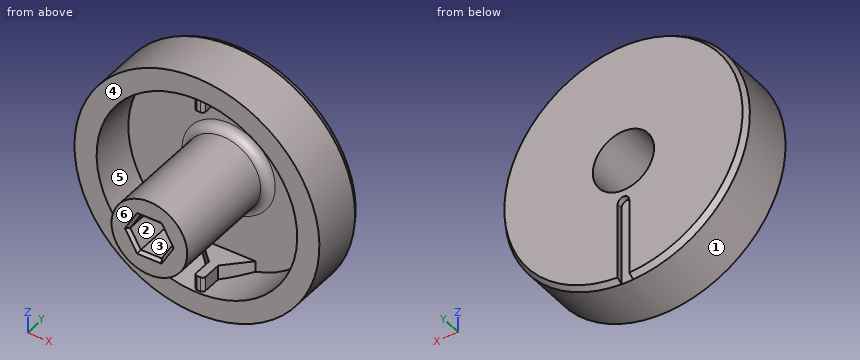
from build123d import *
from build123d.topology import SkipClean

# Parameters (mm, degrees)
SKETCH1_R           = 10.5
SKETCH1_R_2         = 8.6
BOSS_EXTRUDE1_DEPTH = 4
BOSS_EXTRUDE2_DEPTH = 1.25
BOSS_EXTRUDE3_START = 17.2
BOSS_EXTRUDE3_DEPTH = 1.25
BOSS_EXTRUDE4_START = 1
SKETCH3_R           = 10.5
BOSS_EXTRUDE4_DEPTH = 1
SKETCH5_R           = 3.25
BOSS_EXTRUDE5_DEPTH = 10
FILLET2_R           = 0.75
CUT_EXTRUDE1_DEPTH  = 5.25
FILLET1_R           = 0.25
SKETCH7_R           = 2.625
CUT_EXTRUDE2_DEPTH  = 2
CUT_EXTRUDE3_DEPTH  = 0.5
CUT_EXTRUDE4_DEPTH  = 4
CHAMFER2_SIZE       = 0.25
CHAMFER3_SIZE       = 0.5
CHAMFER3_SIZE2      = 0.288675135


with BuildPart() as part:
    # Sketch1 → Boss-Extrude1 (new body)
    with BuildSketch(Plane(origin=(0, 0, 0), x_dir=(1, 0, 0), z_dir=(0, 1, 0))):
        with Locations(Location((0, 0, 0), (0, 0, 270))):
            Circle(SKETCH1_R)
        with Locations(Location((0, 0, 0), (0, 0, 270))):
            Circle(SKETCH1_R_2, mode=Mode.SUBTRACT)
    extrude(amount=-BOSS_EXTRUDE1_DEPTH)

    # Sketch2 → Boss-Extrude2 (add)
    with BuildSketch(Plane(origin=(0, 0, 8.6), x_dir=(-1, 0, 0), z_dir=(0, 0, -1))):
        Polygon((0.4, -3.75), (-0.4, -3.75), (-0.4, -1.9), (-2.3, 0), (2.3, 0), (0.4, -1.9), align=None)
    extrude(amount=BOSS_EXTRUDE2_DEPTH)

    # Sketch2<2> → Boss-Extrude3 (add)
    with BuildSketch(Plane(origin=(0, 0, 8.6), x_dir=(-1, 0, 0), z_dir=(0, 0, -1)).offset(BOSS_EXTRUDE3_START)):
        Polygon((0.4, -3.75), (-0.4, -3.75), (-0.4, -1.9), (-2.3, 0), (2.3, 0), (0.4, -1.9), align=None)
    extrude(amount=-BOSS_EXTRUDE3_DEPTH)

    # Sketch3 → Boss-Extrude4 (add)
    with BuildSketch(Plane(origin=(0, 0, 0), x_dir=(1, 0, 0), z_dir=(0, 1, 0)).offset(BOSS_EXTRUDE4_START)):
        with Locations(Location((0, 0, 0), (0, 0, 270))):
            Circle(SKETCH3_R)
    extrude(amount=-BOSS_EXTRUDE4_DEPTH)

    # Sketch5 → Boss-Extrude5 (add)
    with BuildSketch(Plane.XZ):
        with Locations(Location((0, 0, 0), (0, 0, 90))):
            Circle(SKETCH5_R)
    extrude(amount=BOSS_EXTRUDE5_DEPTH)

    # Fillet2
    fillet2_edges = [part.edges().sort_by_distance(p)[0] for p in [
        (0, 0, -3.25),
    ]]
    fillet(fillet2_edges, radius=FILLET2_R)

    # Sketch4 → Cut-Extrude1 (cut)
    with BuildSketch(Plane(origin=(0, 1, 0), x_dir=(1, 0, 0), z_dir=(0, 1, 0))):
        with BuildLine():
            Line((-1.469693846, 2.175), (1.469693846, 2.175))
            ThreePointArc((1.469693846, 2.175), (0, -2.625), (-1.469693846, 2.175))
        make_face()
    extrude(amount=-CUT_EXTRUDE1_DEPTH, mode=Mode.SUBTRACT)

    # Fillet1
    fillet1_edges = [part.edges().sort_by_distance(p)[0] for p in [
        (-0.4, -3.75, 7.970346319),
        (0.4, -3.75, 7.970346319),
        (-0.4, -3.75, -7.970346319),
        (0.4, -3.75, -7.970346319),
    ]]
    fillet(fillet1_edges, radius=FILLET1_R)

    # Sketch7 → Cut-Extrude2 (cut)
    with SkipClean():  # the faces are left unmerged after this step: merging them gives an invalid solid
        with BuildSketch(Plane(origin=(0, 1, 0), x_dir=(1, 0, 0), z_dir=(0, 1, 0))):
            with Locations(Location((0, 0, 0), (0, 0, 270))):
                Circle(SKETCH7_R)
        extrude(amount=-CUT_EXTRUDE2_DEPTH, mode=Mode.SUBTRACT)

    # Sketch9 → Cut-Extrude3 (cut)
    with SkipClean():  # the faces are left unmerged after this step: merging them gives an invalid solid
        with BuildSketch(Plane(origin=(0, 1, 0), x_dir=(1, 0, 0), z_dir=(0, 1, 0))):
            with BuildLine():
                Line((-0.5, 3.7), (-0.5, 13.7))
                ThreePointArc((-0.5, 13.7), (0, 14.2), (0.5, 13.7))
                Line((0.5, 13.7), (0.5, 3.7))
                ThreePointArc((0.5, 3.7), (0, 3.2), (-0.5, 3.7))
            make_face()
        extrude(amount=-CUT_EXTRUDE3_DEPTH, mode=Mode.SUBTRACT)

    # Sketch10 → Cut-Extrude4 (cut)
    with SkipClean():  # the faces are left unmerged after this step: merging them gives an invalid solid
        with BuildSketch(Plane.XZ.offset(10)):
            Polygon((1.804219591, 0), (0.902109796, 1.5625), (-0.902109796, 1.5625), (-1.804219591, 0), (-0.902109796, -1.5625), (0.902109796, -1.5625), align=None)
        extrude(amount=-CUT_EXTRUDE4_DEPTH, mode=Mode.SUBTRACT)

    # Chamfer2
    chamfer2_edges = [part.edges().sort_by_distance(p)[0] for p in [
        (1.353164693, -10, -0.78125),
        (1.353164693, -10, 0.78125),
        (0, -10, 1.5625),
        (-1.353164693, -10, 0.78125),
        (-1.353164693, -10, -0.78125),
        (0, -10, -1.5625),
    ]]
    chamfer(chamfer2_edges, length=CHAMFER2_SIZE)

    # Chamfer3
    chamfer3_edges = [part.edges().sort_by_distance(p)[0] for p in [
        (-10.497021698, 1, 0.250070932),
    ]]
    chamfer3_side = [part.faces().sort_by_distance(p)[0] for p in [
        (0, -1.5, -10.5),
    ]]
    chamfer(chamfer3_edges, length=CHAMFER3_SIZE, length2=CHAMFER3_SIZE2, reference=chamfer3_side[0])


solid = part.part
Can you work these out from the model? Positions are in its coordinate system, mm. Face numbers are marked on the shaded views. A direction names the side the tool comes from. Coordinates: 2 decimals unless noted, no trailing zeros. Order: outer loops, then holes, each group sorted by start corner. A loop starts at its lowest first (then second) coordinate and runs counter-clockwise, first axis right, second up. Notation, with made-up numbers: (-30.75, -14) - (-9.75, -14) arc R16 ccw to (-9.75, -1) - close; hole circle Ø8 at (71.25, 18.5). An arc over 180 degrees is marked (long way). Answer as a JSON object with one key per item and string values. Group by question number.
Q1. On a 3-axis mill with a long thin cutter (end or side, diameter ignored), from which of +Z, -Z, +X, -X, +Y, -Y can I reach the whole of each face in a straight line? I mean the marked faces 5 and 6. Say none if no direction works.
Q2. Will these pins go through, and if not, where does the flat tip stop? P1, Ø2.5, axis at x = 0, z = 0, coming from the -Y side; P2, Ø0.9, axis at x = -0.5, y = -7.5, coming from the -Z side; P3, Ø0.6, axis at y = 1, z = -6.5, coming from the -X side.
Q3. I need wall thicknesses on line 1 (X direction, y = -2.75, z = 0) (3 decimals); line 2 (X direction, y = -3.25, z = -7.5); line 3 (Y direction, x = 3.5, z = -7.5). Which ranges of each line are inside material? Lowest first, please. Write a range as from..to.
Q4. Imagine slicing it at A-A (y = -8). Please give me the cut outline in (x, z), and give its area (3 significant figures).
Q5. We'd pull the mould along Z, two halves only. Please class the marked faces 1, 2, 3 and 4: +Z half, -Z half, draft (parallel to the pull), parting line (faces both ways), or undercut.
Determined:
{
 "1": {"face 5": "-Y", "face 6": "+Z, -Z, +X, -X, -Y"},
 "2": {"P1": "stops at y = -6", "P2": "stops at z = -3.25", "P3": "stops at x = -8.2"},
 "3": {"line 1": "x = -10.5..-8.6, -3.25..-2.625, 2.625..3.25, 8.6..10.5", "line 2": "x = -7.35..-4.21, -0.4..0.4, 4.21..7.35", "line 3": "y = 0..1"},
 "4": {"outline": "circle Ø6.5 at (0, 0); hole (-1.8, 0) - (-0.9, -1.56) - (0.9, -1.56) - (1.8, 0) - (0.9, 1.56) - (-0.9, 1.56) - close", "area": "24.7 mm2"},
 "5": {"face 1": "parting line", "face 2": "undercut", "face 3": "undercut", "face 4": "draft"}
}
